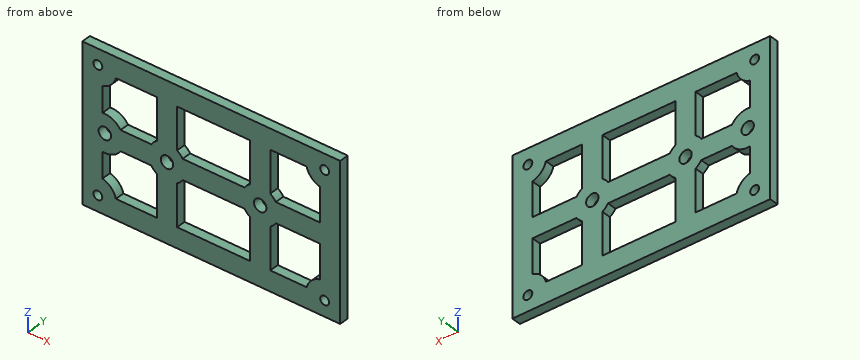
```python
from build123d import *

# Parameters (mm, degrees)
SKETCH1_W            = 83
SKETCH1_H            = 50
BOSS_EXTRUDE1_DEPTH  = 3
SKETCH2_R            = 2
CUT_EXTRUDE1_DEPTH   = 4
SKETCH3_R            = 1.425
CUT_EXTRUDE2_DEPTH   = 4
LPATTERN1_COUNT      = 2
LPATTERN1_PITCH      = 73
LPATTERN1_COUNT_DIR2 = 2
LPATTERN1_PITCH_DIR2 = 40
CUT_EXTRUDE3_DEPTH   = 10


with BuildPart() as part:
    # Sketch1 → Boss-Extrude1 (new body)
    with BuildSketch(Plane(origin=(0, 0, 0), x_dir=(1, 0, 0), z_dir=(0, 1, 0))):
        Rectangle(SKETCH1_W, SKETCH1_H)
    extrude(amount=BOSS_EXTRUDE1_DEPTH)

    # Sketch2 → Cut-Extrude1 (cut, through all)
    with BuildSketch(Plane.XZ):
        with Locations((-34.25, 0)):
            Circle(SKETCH2_R)
        with Locations((-14.25, 0)):
            Circle(SKETCH2_R)
        with Locations((15.75, 0)):
            Circle(SKETCH2_R)
    extrude(amount=-CUT_EXTRUDE1_DEPTH, mode=Mode.SUBTRACT)

    # Sketch3 → Cut-Extrude2 (cut, through all)
    with BuildSketch(Plane.XZ):
        with Locations((-36.5, -20)):
            Circle(SKETCH3_R)
    cut_extrude2 = extrude(amount=-CUT_EXTRUDE2_DEPTH, mode=Mode.SUBTRACT)

    # LPattern1: Cut-Extrude2 2 × 2
    with Locations(*[(i * LPATTERN1_PITCH, 0, j * LPATTERN1_PITCH_DIR2) for i in range(LPATTERN1_COUNT) for j in range(LPATTERN1_COUNT_DIR2) if (i, j) != (0, 0)]):
        add(cut_extrude2, mode=Mode.SUBTRACT)

    # Sketch4 → Cut-Extrude3 (cut)
    with BuildSketch(Plane.XZ):
        with BuildLine():
            Line((0, 18.5), (-11, 18.5))
            Line((-11, 18.5), (-11, 5.04356025))
            ThreePointArc((-11, 5.04356025), (-10.007359313, 4.242640687), (-9.20643975, 3.25))
            Line((-9.20643975, 3.25), (0, 3.25))
            Line((0, 3.25), (10.70643975, 3.25))
            ThreePointArc((10.70643975, 3.25), (11.507359313, 4.242640687), (12.5, 5.04356025))
            Line((12.5, 5.04356025), (12.5, 18.5))
            Line((12.5, 18.5), (0, 18.5))
        make_face()
        with BuildLine():
            Line((0, -3.25), (-9.20643975, -3.25))
            ThreePointArc((-9.20643975, -3.25), (-10.007359313, -4.242640687), (-11, -5.04356025))
            Line((-11, -5.04356025), (-11, -18.5))
            Line((-11, -18.5), (0, -18.5))
            Line((0, -18.5), (12.5, -18.5))
            Line((12.5, -18.5), (12.5, -5.04356025))
            ThreePointArc((12.5, -5.04356025), (11.507359313, -4.242640687), (10.70643975, -3.25))
            Line((10.70643975, -3.25), (0, -3.25))
        make_face()
        with BuildLine():
            Line((-17.5, 18.5), (-30.690524981, 18.5))
            ThreePointArc((-30.690524981, 18.5), (-32.257359313, 15.757359313), (-35, 14.190524981))
            Line((-35, 14.190524981), (-35, 5.95294045))
            ThreePointArc((-35, 5.95294045), (-31.713242882, 5.43735812), (-29.20643975, 3.25))
            Line((-29.20643975, 3.25), (-19.29356025, 3.25))
            ThreePointArc((-19.29356025, 3.25), (-18.492640687, 4.242640687), (-17.5, 5.04356025))
            Line((-17.5, 5.04356025), (-17.5, 18.5))
        make_face()
        with BuildLine():
            Line((-19.29356025, -3.25), (-29.20643975, -3.25))
            ThreePointArc((-29.20643975, -3.25), (-31.713242882, -5.43735812), (-35, -5.95294045))
            Line((-35, -5.95294045), (-35, -14.190524981))
            ThreePointArc((-35, -14.190524981), (-32.257359313, -15.757359313), (-30.690524981, -18.5))
            Line((-30.690524981, -18.5), (-17.5, -18.5))
            Line((-17.5, -18.5), (-17.5, -5.04356025))
            ThreePointArc((-17.5, -5.04356025), (-18.492640687, -4.242640687), (-19.29356025, -3.25))
        make_face()
        with BuildLine():
            Line((20.79356025, 3.25), (35, 3.25))
            Line((35, 3.25), (35, 14.190524981))
            ThreePointArc((35, 14.190524981), (32.257359313, 15.757359313), (30.690524981, 18.5))
            Line((30.690524981, 18.5), (19, 18.5))
            Line((19, 18.5), (19, 5.04356025))
            ThreePointArc((19, 5.04356025), (19.992640687, 4.242640687), (20.79356025, 3.25))
        make_face()
        with BuildLine():
            Line((20.79356025, -3.25), (35, -3.25))
            Line((35, -3.25), (35, -14.190524981))
            ThreePointArc((35, -14.190524981), (32.257359313, -15.757359313), (30.690524981, -18.5))
            Line((30.690524981, -18.5), (19, -18.5))
            Line((19, -18.5), (19, -5.04356025))
            ThreePointArc((19, -5.04356025), (19.992640687, -4.242640687), (20.79356025, -3.25))
        make_face()
    extrude(amount=-CUT_EXTRUDE3_DEPTH, mode=Mode.SUBTRACT)


solid = part.part
```
Read the model definition and answer for the solid it produces. Units are mm, in the model's axes. Give positions to 0.01 mm unless a question says otherwise; leave off trailing zeros. Write each loop counter-clockwise with the first axis right and the second up, starting at its lowest first coordinate (ties: lowest second). Pieces come first, ordered by that corner, then holes. Notation, with made-up numbers: M 24.25,-2 L 69.25,-2 A16 cw 69.25,5 Z; hole C -24,-12 d3. An arc over 180 degrees is marked long. Put each result on its own line as item: value. Start each with the question number.
1. Consider line 1 along X through (y, z) = (1.4, -9); line 2 along Z through (x, y) = (-36.5, 1.95) (3 decimals); line 3 along Z through (x, y) = (24, 2.4). Determine where each line is inside the solid, lowest interval first.
2. The part is cut by section D-D, the plane x = -1.5. Give the vertices of the cut face in (y, z), and give its area (3 significant figures).
3. The part is cut by section C-C, the plane z = 0. Give the vertices of the cut face in (x, y).
4. This flat-tipped pin is pushed along its axis until it touches: pin 1 Ø2.5 at (x, z) = (-34.25, 0) entering from +Y. Where does it stop, or does it pass through?
5. The part is cut by section A-A, the plane z = -20. Give the vertices of the cut face in (x, y) (3 decimals).
6. The part is cut by section B-B, the plane x = -14.25. Give the vertices of the cut face in (y, z), and give its area (3 significant figures).
Final values:
1. line 1: x = -41.5 to -35, -17.5 to -11, 12.5 to 19, 35 to 41.5
1. line 2: z = -25 to -21.425, -18.575 to 18.575, 21.425 to 25
1. line 3: z = -25 to -18.5, -3.25 to 3.25, 18.5 to 25
2. outline: M 0,-25 L 3,-25 L 3,-18.5 L 0,-18.5 Z; M 0,-3.25 L 3,-3.25 L 3,3.25 L 0,3.25 Z; M 0,18.5 L 3,18.5 L 3,25 L 0,25 Z
2. area: 58.5 mm²
3. outline: M -41.5,0 L -36.25,0 L -36.25,3 L -41.5,3 Z; M -32.25,0 L -16.25,0 L -16.25,3 L -32.25,3 Z; M -12.25,0 L 13.75,0 L 13.75,3 L -12.25,3 Z; M 17.75,0 L 41.5,0 L 41.5,3 L 17.75,3 Z
4. pin 1: passes through
5. outline: M -41.5,0 L -37.925,0 L -37.925,3 L -41.5,3 Z; M -35.075,0 L 35.075,0 L 35.075,3 L -35.075,3 Z; M 37.925,0 L 41.5,0 L 41.5,3 L 37.925,3 Z
6. outline: M 0,-25 L 3,-25 L 3,-2 L 0,-2 Z; M 0,2 L 3,2 L 3,25 L 0,25 Z
6. area: 138 mm²
